Model file for the job. Use its own axes, mm. Give positions to 0.01 mm unless a question says otherwise; leave off trailing zeros. Loops run counter-clockwise (first coordinate to the right, second up) from the corner with the lowest first, then second, coordinate; pieces in that order, holes last. Notation, with made-up numbers: (-26, -26.5) - (32, -26.5) arc R36 cw to (32, 7.5) - close; hole circle Ø8 at (-37, -18.5). An arc over 180 degrees is marked (long way). Use a Markdown table: item, result.
from build123d import *

# Parameters (mm, degrees)
CROQUIS1_R              = 55
SALIENTE_EXTRUIR1_DEPTH = 5
CORTAR_EXTRUIR1_DEPTH   = 78.942286341
CROQUIS3_R              = 2
CORTAR_EXTRUIR2_DEPTH   = 10
CROQUIS4_R              = 25
CORTAR_EXTRUIR3_DEPTH   = 78.942286341


with BuildPart() as part:
    # Croquis1 → Saliente-Extruir1 (new body)
    with BuildSketch(Plane.XY):
        Circle(CROQUIS1_R)
    extrude(amount=SALIENTE_EXTRUIR1_DEPTH)

    # Croquis2 → Cortar-Extruir1 (cut, through all)
    with BuildSketch(Plane.XY.offset(5)):
        Polygon((-21.161601507, 50.8315113), (-16.031299357, 36.736121988), (-11.332836253, 38.446222705), (-16.463138403, 52.541612016), align=None)
        Polygon((16.031299357, 36.736121988), (11.332836253, 38.446222705), (16.463138403, 52.541612016), (21.161601507, 50.8315113), align=None)
        Polygon((54.602180852, -7.08927116), (39.830064557, -4.484548495), (38.961823668, -9.40858726), (53.733939964, -12.013309925), align=None)
        Polygon((27.628987415, -29.037635445), (37.27080156, -40.528302091), (33.440579345, -43.74224014), (23.7987652, -32.251573493), align=None)
        Polygon((-33.440579345, -43.74224014), (-23.7987652, -32.251573493), (-27.628987415, -29.037635445), (-37.27080156, -40.528302091), align=None)
        Polygon((-38.961823668, -9.40858726), (-53.733939964, -12.013309925), (-54.602180852, -7.08927116), (-39.830064557, -4.484548495), align=None)
    extrude(amount=-CORTAR_EXTRUIR1_DEPTH, mode=Mode.SUBTRACT)

    # Croquis3 → Cortar-Extruir2 (cut)
    with BuildSketch(Plane.XY.offset(5)):
        with Locations((0, 45)):
            Circle(CROQUIS3_R)
        with Locations((0, -45)):
            Circle(CROQUIS3_R)
        with Locations((38.97114317, -22.5)):
            Circle(CROQUIS3_R)
        with Locations((-38.97114317, 22.5)):
            Circle(CROQUIS3_R)
        with Locations((-38.97114317, -22.5)):
            Circle(CROQUIS3_R)
        with Locations((38.97114317, 22.5)):
            Circle(CROQUIS3_R)
    extrude(amount=-CORTAR_EXTRUIR2_DEPTH, mode=Mode.SUBTRACT)

    # Croquis4 → Cortar-Extruir3 (cut, through all)
    with BuildSketch(Plane(origin=(0, 0, 0), x_dir=(-1, 0, 0), z_dir=(0, 0, -1))):
        Circle(CROQUIS4_R)
    extrude(amount=-CORTAR_EXTRUIR3_DEPTH, mode=Mode.SUBTRACT)


solid = part.part
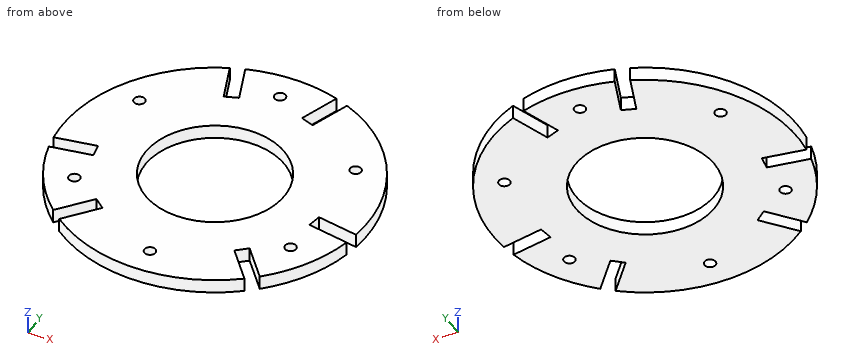
(1) Pin check, flat tips, straight feed: P1, Ø3, axis at x = -20.5, y = 41.5, coming from the -Z side; P2, Ø3, axis at y = 30.5, z = 1.5, coming from the +X side; P3, Ø1, axis at x = 0, z = 3, coming from the +Y side; P4, Ø2, axis at y = 21.5, z = 2, coming from the -X side. Stop position of each tip, or through.
Computed:
| item | result |
|---|---|
| P1 | z = 0 |
| P2 | x = 46.73 |
| P3 | y = 55 |
| P4 | x = -51.04 |
(2) Slice it at A-A, the plane y = 0. Write the cut outline in (x, z).
Computed:
| item | result |
|---|---|
| outline | (-55, 0) - (-25, 0) - (-25, 5) - (-55, 5) - close; (25, 0) - (55, 0) - (55, 5) - (25, 5) - close |
(3) Drill centre lines: probe 1 along Y at (x, z) = (9.5, 1.25); probe 2 along X at (y, z) = (6, 4.6); probe 3 along Y at (x, z) = (-11, 0.3). Where is each one in solid material? Low to high. Write a range as [from, to].
Computed:
| item | result |
|---|---|
| probe 1 | [-54.17, -23.12], [23.12, 54.17] |
| probe 2 | [-54.67, -24.27], [24.27, 54.67] |
| probe 3 | [-53.89, -22.45], [22.45, 53.89] |
(4) Slice it at D-D, the plane y = 45. Write the cut outline in (x, z), plus the area to 3 significant figures.
Computed:
| item | result |
|---|---|
| outline | (-31.62, 0) - (-19.04, 0) - (-19.04, 5) - (-31.62, 5) - close; (-13.72, 0) - (-2, 0) - (-2, 5) - (-13.72, 5) - close; (2, 0) - (13.72, 0) - (13.72, 5) - (2, 5) - close; (19.04, 0) - (31.62, 0) - (31.62, 5) - (19.04, 5) - close |
| area | 243 mm² |
(5) Slice it at C-C, the plane z = 3.2. Count the separate pieces of the cut face and the enclosed holes in it, plus the area to 3 significant figures.
Computed:
| item | result |
|---|---|
| separate pieces | 1 |
| enclosed holes | 7 |
| area | 7,020 mm² |
(6) Slice it at B-B, the plane x = 0. Write the cut outline in (y, z).
Computed:
| item | result |
|---|---|
| outline | (-55, 0) - (-47, 0) - (-47, 5) - (-55, 5) - close; (-43, 0) - (-25, 0) - (-25, 5) - (-43, 5) - close; (25, 0) - (43, 0) - (43, 5) - (25, 5) - close; (47, 0) - (55, 0) - (55, 5) - (47, 5) - close |
